Geometry check sheet. Reference: the model listing, model coordinates, mm. Give positions to 0.01 mm unless a question says otherwise; leave off trailing zeros. Loops run counter-clockwise (first coordinate to the right, second up) from the corner with the lowest first, then second, coordinate; pieces in that order, holes last. Notation, with made-up numbers: (-23, 80) - (4, 80) arc R3 ccw to (4, 85) - close; hole circle Ø8 at (60.25, 87.25). An arc over 180 degrees is marked (long way). Use a Markdown table: item, result. Add a question column.
1. Cross-section at D-D on z = 19. Enter the section's corners in (x, y).
2. Material ranges on L1, parallel to X at y = 1.35, z = 183; L2, parallel to X at y = 1.55, z = -5; L3, parallel to Z at x = 137, y = 3.6, recorded low to high.
3. Cross-section at A-A on x = 244. Enter the section's corners in (y, z), and give its area (3 significant figures).
4. Cross-section at C-C on z = 85. Enter the section's corners in (x, y), and give its area (3 significant figures).
5. Depth check by flat-ended pin: P1, Ø2, axis at y = 2.5, z = 41.5, coming from the +X side; P2, Ø3, axis at x = 135.5, y = 2.5, coming from the -Z side; P3, Ø1.5, axis at y = 3, z = 134.5, coming from the +X side. Enter the tip coordinate at first touch or a pass-through.
6. Cross-section at B-B on y = 3.7. Count the separate pieces of the cut face and the enclosed holes in it, and give its area (3 significant figures).
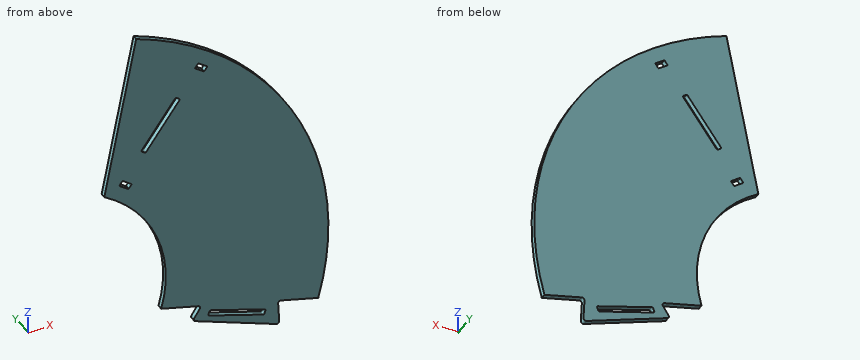
Autodesk Inventor part; units mm, degrees
ref_plane "YZ Plane" through (0, 0, 0) normal (1, 0, 0) x (0, 1, 0)
ref_plane "XZ Plane" through (0, 0, 0) normal (0, 1, 0) x (-1, 0, 0)
ref_plane "XY Plane" through (0, 0, 0) normal (0, 0, 1) x (1, 0, 0)
sketch "Sketch1" plane through (0, 0, 0) normal (0, 1, 0) x (-1, 0, 0)
  circle A0 centre (0, 0) radius 341.36
  circle A1 centre (0, 0) radius 150.07
  dimension "d84" = 300.14
  dimension "d85" = 682.72
extrude "Extrusion3" add sketch "Sketch1" along normal blind 6 contours A0 | A1
sketch "Sketch2" plane through (0, 6, 0) normal (0, 1, 0) x (1, 0, 0)
  circle A0 centre (0, 0) radius 245.715 construction
  line L0 (245.7148, 0.3131) -> (341.6521, -0.0088)
  line L1 (3.25, 279.0483) -> (3.25, 212.3817)
  line L2 (-3.25, 212.3817) -> (-3.25, 279.0483)
  arc A1 (-3.25, 212.3817) -> (-1.9167, 211.0483) centre (-1.9167, 212.3817) ccw
  arc A2 (1.9167, 211.0483) -> (3.25, 212.3817) centre (1.9167, 212.3817) ccw
  arc A3 (-1.9167, 280.3817) -> (-3.25, 279.0483) centre (-1.9167, 279.0483) ccw
  arc A4 (3.25, 279.0483) -> (1.9167, 280.3817) centre (1.9167, 279.0483) ccw
  line L3 (-1.9167, 280.3817) -> (1.9167, 280.3817)
  line L4 (-1.9167, 211.0483) -> (1.9167, 211.0483)
  line L5 (0, 0) -> (0, 212.3817)
  line L6 (0, 280.3817) -> (0, 341.36)
  line L7 (0, 211.0483) -> (0, 245.715) construction
  line L8 (0, 280.3817) -> (0, 245.715) construction
  line L9 (-266.6835, 86.5666) -> (-233.7136, 75.854) construction
  line L10 (-264.4112, 89.2455) -> (-201.0074, 68.6444)
  arc A5 (-200.1513, 66.9643) -> (-201.0074, 68.6444) centre (-201.4194, 67.3763) ccw
  line L11 (-200.7436, 65.1414) -> (-233.7136, 75.854) construction
  line L12 (-201.3359, 63.3186) -> (-200.1513, 66.9643)
  line L13 (-267.2758, 84.7438) -> (-266.0912, 88.3895)
  line L14 (-203.016, 62.4625) -> (-266.4198, 83.0637)
  arc A6 (-203.016, 62.4625) -> (-201.3359, 63.3186) centre (-202.604, 63.7306) ccw
  arc A7 (-267.2758, 84.7438) -> (-266.4198, 83.0637) centre (-266.0077, 84.3317) ccw
  arc A8 (-264.4112, 89.2455) -> (-266.0912, 88.3895) centre (-264.8232, 87.9775) ccw
  line L15 (-165.0631, -226.6454) -> (-144.6865, -198.5995) construction
  line L16 (-166.9087, -223.6565) -> (-127.723, -169.722)
  arc A9 (-125.8606, -169.427) -> (-127.723, -169.722) centre (-126.6443, -170.5057) ccw
  line L17 (-124.31, -170.5536) -> (-144.6865, -198.5995) construction
  line L18 (-122.7594, -171.6802) -> (-125.8606, -169.427)
  line L19 (-163.5125, -227.772) -> (-166.6137, -225.5189)
  line L20 (-122.4644, -173.5426) -> (-161.6501, -227.4771)
  arc A10 (-122.4644, -173.5426) -> (-122.7594, -171.6802) centre (-123.5431, -172.7589) ccw
  arc A11 (-163.5125, -227.772) -> (-161.6501, -227.4771) centre (-162.7288, -226.6933) ccw
  arc A12 (-166.9087, -223.6565) -> (-166.6137, -225.5189) centre (-165.83, -224.4402) ccw
  line L21 (164.8042, -226.8335) -> (144.4277, -198.7876) construction
  line L22 (160.9139, -228.0119) -> (121.7282, -174.0775)
  arc A13 (122.0232, -172.2151) -> (121.7282, -174.0775) centre (122.8069, -173.2938) ccw
  line L23 (123.5738, -171.0885) -> (144.4277, -198.7876) construction
  line L24 (125.1244, -169.9619) -> (122.0232, -172.2151)
  line L25 (165.8775, -226.0537) -> (162.7763, -228.3069)
  line L26 (126.9868, -170.2569) -> (166.1725, -224.1913)
  arc A14 (126.9868, -170.2569) -> (125.1244, -169.9619) centre (125.9081, -171.0406) ccw
  arc A15 (165.8775, -226.0537) -> (166.1725, -224.1913) centre (165.0938, -224.975) ccw
  arc A16 (160.9139, -228.0119) -> (162.7763, -228.3069) centre (161.9926, -227.2282) ccw
  line L27 (266.7793, 86.2718) -> (233.8094, 75.5592) construction
  line L28 (266.5156, 82.7688) -> (203.1118, 62.1677)
  arc A17 (201.4317, 63.0238) -> (203.1118, 62.1677) centre (202.6998, 63.4358) ccw
  line L29 (200.8394, 64.8466) -> (233.8094, 75.5592) construction
  line L30 (200.2471, 66.6695) -> (201.4317, 63.0238)
  line L31 (266.187, 88.0946) -> (267.3716, 84.4489)
  line L32 (201.1032, 68.3496) -> (264.5069, 88.9507)
  arc A18 (201.1032, 68.3496) -> (200.2471, 66.6695) centre (201.5152, 67.0815) ccw
  arc A19 (266.187, 88.0946) -> (264.5069, 88.9507) centre (264.919, 87.6826) ccw
  arc A20 (266.5156, 82.7688) -> (267.3716, 84.4489) centre (266.1035, 84.0369) ccw
  point P0 (-202.0117, 65.5535)
  point P1 (-125.0937, -171.6323)
  point P2 (124.8348, -171.8204)
  point P3 (202.1075, 65.2586)
  dimension "d21" = 6.5
  dimension "d24" = 2.6667
  dimension "d25" = 2.6667
  dimension "d32" = 1.3333
  dimension "d33" = 1.3333
  dimension "d41" = 90
  dimension "d42" = 3.25
  dimension "d43" = 90
  dimension "d86" = 491.43
extrude "Extrusion4" cut sketch "Sketch2" against normal through all
sketch "Sketch3" plane through (0, 6, 0) normal (0, 1, 0) x (1, 0, 0)
  arc A0 (-115.2299, -321.3234) -> (115.2355, -321.3214) centre (0, 0) ccw
  arc A1 (-77.7244, -128.3741) -> (77.7297, -128.3709) centre (0, 0) ccw
  line L0 (-122.1811, -173.696) -> (-161.3589, -227.6196)
  line L1 (-115.2299, -321.3234) -> (-77.7244, -128.3741)
  line L2 (0, 0) -> (0, -341.2918)
  line L3 (115.2355, -321.3214) -> (77.7297, -128.3709)
  line L4 (161.3912, -227.6651) -> (122.2055, -173.7307)
  dimension "d52" = 25
  dimension "d87" = 150.07
  dimension "d88" = 341.36
  dimension "d89" = 25
  dimension "d90" = 11
  dimension "d91" = 11
extrude "Extrusion5" cut sketch "Sketch3" against normal blind 10
sketch "Sketch5" plane through (0, 6, 0) normal (0, 1, 0) x (1, 0, 0)
  line L0 (3.25, 279.0483) -> (3.25, 212.3817)
  line L1 (5.5862, 197.9634) -> (-6.155, 194.8174)
  line L2 (-11.2263, 301.7146) -> (10.5847, 293.3421)
  line L3 (6.5657, 149.9554) -> (8.9394, 195.248)
  line L4 (14.2034, 295.6921) -> (16.5771, 340.9846)
  arc A0 (10.5847, 293.3421) -> (14.2034, 295.6921) centre (11.5404, 295.8316) ccw
  arc A1 (8.9394, 195.248) -> (5.5862, 197.9634) centre (6.2763, 195.3876) ccw
  arc A2 (-11.2263, 301.7146) -> (-14.8449, 299.0854) centre (-12.1819, 299.225) ccw
  line L5 (-3.25, 212.3817) -> (-3.25, 279.0483)
  line L6 (-14.8449, 299.0854) -> (-9.5081, 197.2536)
  arc A3 (-9.5081, 197.2536) -> (-6.155, 194.8174) centre (-6.8451, 197.3932) ccw
  line L7 (-1.9167, 211.0483) -> (1.9167, 211.0483)
  line L8 (1.9167, 280.3817) -> (-1.9167, 280.3817)
  arc A4 (115.2355, -321.3214) -> (-115.2299, -321.3234) centre (0, 0) ccw
  line L9 (16.5771, 340.9846) -> (16.5774, 340.9903)
  arc A5 (-190.5375, 51.9119) -> (-187.1843, 54.3482) centre (-189.8473, 54.4877) ccw
  line L10 (-186.5481, 66.4868) -> (-187.1843, 54.3482)
  arc A6 (-182.9295, 68.8368) -> (-186.5481, 66.4868) centre (-183.8851, 66.3472) ccw
  arc A7 (-275.714, 100.7144) -> (-276.8308, 104.8821) centre (-277.7864, 102.3926) ccw
  line L11 (-289.0345, 78.3041) -> (-190.5375, 51.9119)
  arc A8 (-290.4167, 82.5581) -> (-289.0345, 78.3041) centre (-288.3443, 80.8799) ccw
  line L12 (-290.4167, 82.5581) -> (-275.714, 100.7144)
  line L13 (-276.8308, 104.8821) -> (-319.1731, 121.1358)
  line L14 (-140.5872, 52.5831) -> (-182.9295, 68.8368)
  line L15 (-319.1731, 121.1358) -> (-319.1784, 121.1378)
  arc A9 (184.6611, 69.9975) -> (183.3803, 66.0556) centre (185.6168, 67.508) ccw
  line L16 (190.0006, 55.8613) -> (183.3803, 66.0556)
  arc A10 (188.4543, 51.8331) -> (190.0006, 55.8613) centre (187.7641, 54.4089) ccw
  arc A11 (282.2558, 80.581) -> (285.609, 77.8656) centre (284.9188, 80.4414) ccw
  line L17 (279.8598, 106.5409) -> (184.6611, 69.9975)
  arc A12 (283.4785, 103.9117) -> (279.8598, 106.5409) centre (280.8155, 104.0513) ccw
  line L18 (283.4785, 103.9117) -> (282.2558, 80.581)
  line L19 (285.609, 77.8656) -> (329.4183, 89.6043)
  line L20 (144.645, 40.0945) -> (188.4543, 51.8331)
  line L21 (329.4183, 89.6043) -> (329.4238, 89.6058)
  circle A13 centre (0, 0) radius 150.07
  line L22 (-140.5872, 52.5831) -> (-140.5479, 52.568)
  line L23 (144.645, 40.0945) -> (144.5122, 40.0589)
  line L24 (6.5657, 149.9554) -> (6.5621, 149.8874)
  arc A14 (-77.7244, -128.3741) -> (77.7297, -128.3709) centre (0, 0) ccw
  arc A15 (115.2355, -321.3214) -> (-115.2299, -321.3234) centre (0, 0) ccw
  line L25 (77.7297, -128.3709) -> (115.2355, -321.3214)
  line L26 (-77.7244, -128.3741) -> (-115.2299, -321.3234)
  point P0 (-77.7399, -128.3998)
  point P1 (77.7399, -128.3998)
  point P2 (-319.1475, 121.126)
  point P3 (-140.56, 52.5727)
  point P4 (6.5642, 149.9264)
  point P5 (16.5757, 340.9573)
  point P6 (329.3918, 89.5972)
  point P7 (144.6169, 40.0869)
  dimension "d63" = 2.6667
  dimension "d64" = 3
  dimension "d66" = 3
  dimension "d67" = 2.6667
  dimension "d68" = 2.6667
  dimension "d70" = 72
  dimension "d71" = 72
  dimension "d94" = 300.14
  dimension "d95" = 682.72
sketch "Sketch6" plane through (0, 6, 0) normal (0, 1, 0) x (1, 0, 0)
  line L0 (188.7727, -264.2184) -> (198.4809, -257.165)
  line L1 (194.6603, -251.9064) -> (184.9521, -258.9598)
  line L2 (161.3912, -227.6651) -> (122.2055, -173.7307)
  line L3 (166.3548, -225.7069) -> (163.2536, -227.9601)
  arc A0 (195.5915, -252.0539) -> (194.6603, -251.9064) centre (195.0522, -252.4457) ccw
  arc A1 (198.4809, -257.165) -> (198.6284, -256.2338) centre (198.0891, -256.6256) ccw
  arc A2 (187.8415, -264.0709) -> (188.7727, -264.2184) centre (188.3809, -263.6791) ccw
  arc A3 (184.9521, -258.9598) -> (184.8046, -259.891) centre (185.344, -259.4991) ccw
  line L4 (184.8046, -259.891) -> (187.8415, -264.0709)
  line L5 (198.6284, -256.2338) -> (195.5915, -252.0539)
  line L6 (122.2055, -173.7307) -> (161.3912, -227.6651)
  line L7 (141.7983, -200.6979) -> (147.057, -196.8773)
  line L8 (166.6498, -223.8445) -> (127.4641, -169.9101)
  line L9 (95.9027, -136.3937) -> (105.6109, -129.3403)
  line L10 (109.4315, -134.5989) -> (99.7233, -141.6523)
  arc A4 (109.4315, -134.5989) -> (109.579, -133.6677) centre (109.0396, -134.0596) ccw
  arc A5 (106.5421, -129.4878) -> (105.6109, -129.3403) centre (106.0027, -129.8796) ccw
  arc A6 (95.9027, -136.3937) -> (95.7552, -137.3249) centre (96.2945, -136.9331) ccw
  arc A7 (98.7921, -141.5048) -> (99.7233, -141.6523) centre (99.3314, -141.113) ccw
  line L11 (98.7921, -141.5048) -> (95.7552, -137.3249)
  line L12 (106.5421, -129.4878) -> (109.579, -133.6677)
  point P0 (0, 0)
  dimension "d104" = 6.5
  dimension "d105" = 12
  dimension "d108" = 1.3333
  dimension "d109" = 1.3333
  dimension "d110" = 1.3333
  dimension "d111" = 1.3333
  dimension "d112" = 0
  dimension "d149" = 145
  dimension "d150" = 90
  dimension "d151" = 90
  dimension "d152" = 90
  dimension "d153" = 90
extrude "Extrusion7" cut sketch "Sketch6" against normal through all
pattern_circular "Circular Pattern2" count 2 over 72 about axis through (0, -10, 0) along (0, 1, 0) of "Extrusion7"
pattern_circular "Circular Pattern3" count 2 over 144 about axis through (0, -10, 0) along (0, 1, 0) of "Extrusion7"
mirror "Mirror3" about plane through (0, 0, 0) normal (1, 0, 0) of "Extrusion7"
pattern_circular "Circular Pattern4" count 2 over 144 about axis through (0, -10, 0) along (0, -1, 0) of "Extrusion7"
extrude "Extrusion10" cut sketch "Sketch5" against normal through all contours A1 L3 L24 A13 L22 L14 A6 L10 A5 L11 A8 L12 A7 L13 A4 L4 A0 L2 A2 L6 A3 L1 | L1 A3 L6 A2 L2 A0 L4 A4 L19 A11 L18 A12 L17 A9 L16 A10 L20 L23 A13 L24 L3 A1 | A13 | A13 L26 A4 L13 A7 L12 A8 L11 A5 L10 A6 L14 L22
equation "\"BendRadius\" = Thickness"
equation "\"BendReliefWidth\" = Thickness"
equation "\"BendReliefDepth\" = 0.5 * Thickness"
equation "\"CornerReliefSize\" = 4 * Thickness"
equation "\"MinimumRemnant\" = 2 * Thickness"
equation "\"TransitionRadius\" = BendRadius"
equation "\"JacobiRadiusSize\" = BendRadius"
equation "\"GapSize\" = Thickness"
properties part number "Ring D4" material "Wood (Maple)"
Values found:
| question | item | result |
|---|---|---|
| 1 | outline | (148.86, 0) - (340.83, 0) - (340.83, 6) - (148.86, 6) - close |
| 2 | L1 | x = 88.35 to 128.21, 136.25 to 288.16 |
| 2 | L2 | x = 149.99 to 341.32 |
| 2 | L3 | z = 61.25 to 184.04, 195.1 to 312.66 |
| 3 | outline | (0, -92.78) - (6, -92.78) - (6, -82.29) - (0, -82.29) - close; (0, -75.45) - (6, -75.45) - (6, 238.73) - (0, 238.73) - close |
| 3 | area | 1,950 mm2 |
| 4 | outline | (123.68, 0) - (330.61, 0) - (330.61, 6) - (123.68, 6) - close |
| 4 | area | 1,240 mm2 |
| 5 | P1 | stops at x = 338.95 |
| 5 | P2 | stops at z = 61.25 |
| 5 | P3 | stops at x = 314.07 |
| 6 | separate pieces | 1 |
| 6 | enclosed holes | 4 |
| 6 | area | 68,700 mm2 |
